Autodesk Inventor part; units mm, degrees
ref_plane "YZ Plane" through (0, 0, 0) normal (1, 0, 0) x (0, 1, 0)
ref_plane "XZ Plane" through (0, 0, 0) normal (0, 1, 0) x (-1, 0, 0)
ref_plane "XY Plane" through (0, 0, 0) normal (0, 0, 1) x (1, 0, 0)
sketch "Sketch1" plane through (0, 0, 0) normal (0, 1, 0) x (-1, 0, 0)
  circle A0 centre (0, 0) radius 5
  dimension "d0" = 10
extrude "Extrusion1" add sketch "Sketch1" along normal blind 10
sketch "Sketch2" plane through (0, 10, 0) normal (0, 1, 0) x (1, 0, 0)
  circle A0 centre (0, 0) radius 1.5
  dimension "d3" = 3
extrude "Extrusion2" add sketch "Sketch2" along normal blind 5
sketch "Sketch3" plane through (0, 0, 0) normal (0, -1, 0) x (1, 0, 0)
  circle A0 centre (0, 0) radius 3
  dimension "d6" = 6
hole "Hole1" at (0, 0, 0) direction (0, 1, 0) diameter 6.5 depth 7
properties part number "acople2"
Geometry: final body of the model. Coordinates: model frame, mm. A direction names the side the tool comes from. Round coordinates to 2 decimals unless told otherwise and drop trailing zeros. Order: outer loops, then holes, each group sorted by start corner. A loop starts at its lowest first (then second) coordinate and runs counter-clockwise, first axis right, second up. Notation, with made-up numbers: (18.5, 18) -> (31.5, 18) arc R35 ccw to (31.5, 50) -> close; hole circle Ø6 at (56.25, 44). An arc over 180 degrees is marked (long way). Use one line per item in the form item = value. Start each with the question number.
1. Draft query along X for faces 4 (the face through (1.08, 4.93, 4.88)), 5 (the face through (1.2, 10, 1.2)), 6 (the face through (1.978, 3.549, 2.579)). Return one class per face: pulls with the +X half, pulls with the -X half, needs draft (parallel to the pull), parting line crosses it, or undercut.
2. Cut plane C-C (z = 0). Return the cut outline in (x, y).
3. Line query: probe 1 along Z at (x, y) = (0, 5.25); probe 2 along Y at (x, z) = (4, -1.25); probe 3 along Y at (x, z) = (0.5, 2.5). Output: solid intervals per line, ascending.
4. Reachability of faces 1 (the face through (-1.5, 12.46, 0.07)), 2 (the face through (-3.3, 0, -1)), 3 (the face through (0, 7, 0)) from +Z, -Z, +X, -X, +Y, -Y: full face, straight path, thin tool, end or side. Return the list, or none.
5. Cut plane B-B (y = 5.25). Return the cut outline in (x, z).
6. Cut plane A-A (x = 0). Return the cut outline in (y, z).
7. Cut plane D-D (x = 3). Return the cut outline in (y, z).
8. Pin query (flat end, axial travel): pin 1 Ø1.5 at (x, z) = (-4, 3.5) entering from +Y; pin 2 Ø5 at (y, z) = (13, -2) entering from -X. Return the tip coordinate at first contact, or that it passes through.
Solution:
q1.face_4 = parting line crosses it
q1.face_5 = needs draft
q1.face_6 = undercut
q2.outline = (-5, 0) -> (-3.25, 0) -> (-3.25, 7) -> (3.25, 7) -> (3.25, 0) -> (5, 0) -> (5, 10) -> (1.5, 10) -> (1.5, 15) -> (-1.5, 15) -> (-1.5, 10) -> (-5, 10) -> close
q3.probe_1 = -5 to -3.25, 3.25 to 5
q3.probe_2 = 0 to 10
q3.probe_3 = 7 to 10
q4.face_1 = +Y
q4.face_2 = +Z, -Z, +X, -X, -Y
q4.face_3 = -Y
q5.outline = circle Ø10 at (0, 0); hole circle Ø6.5 at (0, 0)
q6.outline = (0, -5) -> (10, -5) -> (10, -1.5) -> (15, -1.5) -> (15, 1.5) -> (10, 1.5) -> (10, 5) -> (0, 5) -> (0, 3.25) -> (7, 3.25) -> (7, -3.25) -> (0, -3.25) -> close
q7.outline = (0, -4) -> (10, -4) -> (10, 4) -> (0, 4) -> (0, 1.25) -> (7, 1.25) -> (7, -1.25) -> (0, -1.25) -> close
q8.pin_1 = 10
q8.pin_2 = -1.5
